Read the model definition and answer for the solid it produces. Units are mm, in the model's axes. A direction names the side the tool comes from. Give positions to 0.01 mm unless a question says otherwise; leave off trailing zeros. Order: outer loops, then holes, each group sorted by start corner. A loop starts at its lowest first (then second) coordinate and runs counter-clockwise, first axis right, second up. Notation, with made-up numbers: (58.5, 39.25) -> (111.5, 39.25) arc R31 ccw to (111.5, 71.25) -> close; hole circle Ø7 at (24, 57.25). An arc over 180 degrees is marked (long way). Answer as CSV lines item,"result". Start each with the question number.
1) The mould has two halves that part along Z. Classify faces 3 (the face through (9, 561, -218.338)), 4 (the face through (0, 295, -182)), 5 (the face through (9, 173, 0)): +Z half, -Z half, draft (parallel to the pull), parting line (faces both ways), or undercut.
2) Find section C-C (y = 425). Determine the outline of the cut face in (x, z), and give its area (3 significant figures).
3) Find section B-B (z = -304.5). Determine the outline of the cut face in (x, y).
4) Straight lines are drawn through the part: L1, parallel to Z at x = 15.5, y = 241.5; L2, parallel to Z at x = 5.75, y = 555; L3, parallel to Z at x = 5.5, y = 254. For each, find the intervals that lie inside material, in ascending order. Write a range as from..to.
5) Flat-ended cylindrical pins translate along their axes: pin 1 Ø5 at (x, y) = (13, 566) entering from +Z; pin 2 Ø1.5 at (x, y) = (15, 448) entering from -Z. Find the tip coordinate at first contact, or state that the pin passes through.
6) For faces 1 (the face through (9, 119, -368.3)), 2 (the face through (9, 562, -151.663)), determine the directions among +Z, -Z, +X, -X, +Y, -Y from which every point of the face is accessible in a straight line to the end or side of a thin tool.
7) Find section A-A (x = 5). Determine the outline of the cut face in (y, z) (1 decimal).
```python
from build123d import *

# Parameters (mm, degrees)
BOSS_EXTRUDE1_DEPTH = 17.4625
CUT_EXTRUDE1_DEPTH  = 17.4625
SKETCH2_R           = 3.96875
CUT_EXTRUDE2_DEPTH  = 17.4625


with BuildPart() as part:
    # Sketch1 → Boss-Extrude1 (new body)
    with BuildSketch(Plane(origin=(0, 0, 0), x_dir=(0, 0, -1), z_dir=(1, 0, 0))):
        Polygon((0, 0), (368.3, 0), (368.3, 241.3), (289.73584427, 581.598745126), (80.26426737, 581.598745126), (0, 340.614), align=None)
    extrude(amount=BOSS_EXTRUDE1_DEPTH)

    # RockerBoxCutout → Cut-Extrude1 (cut)
    with BuildSketch(Plane(origin=(17.4625, 0, 0), x_dir=(0, 0, -1), z_dir=(1, 0, 0))):
        with BuildLine():
            ThreePointArc((218.33755582, 541.911245126), (185.00005582, 575.248745126), (151.66255582, 541.911245126))
            Line((151.66255582, 541.911245126), (218.33755582, 541.911245126))
        make_face()
        with BuildLine():
            Line((218.33755582, 541.911245126), (151.66255582, 541.911245126))
            ThreePointArc((151.66255582, 541.911245126), (185.00005582, 508.573745126), (218.33755582, 541.911245126))
        make_face()
        with BuildLine():
            Line((151.66255582, 581.598745126), (151.66255582, 541.911245126))
            ThreePointArc((151.66255582, 541.911245126), (185.00005582, 575.248745126), (218.33755582, 541.911245126))
            Line((218.33755582, 541.911245126), (218.33755582, 581.598745126))
            Line((218.33755582, 581.598745126), (151.66255582, 581.598745126))
        make_face()
    extrude(amount=-CUT_EXTRUDE1_DEPTH, mode=Mode.SUBTRACT)

    # Sketch2 → Cut-Extrude2 (cut)
    with BuildSketch(Plane.ZY):
        with Locations((-13, 60)):
            Circle(SKETCH2_R)
        with Locations((-13, 290.1875)):
            Circle(SKETCH2_R)
    extrude(amount=-CUT_EXTRUDE2_DEPTH, mode=Mode.SUBTRACT)


solid = part.part
```
Findings below:
1,face 3,"undercut"
1,face 4,"draft"
1,face 5,"+Z half"
2,outline,"(0, -325.89) -> (17.46, -325.89) -> (17.46, -28.11) -> (0, -28.11) -> close"
2,area,"5,200 mm²"
3,outline,"(0, 0) -> (17.46, 0) -> (17.46, 517.65) -> (0, 517.65) -> close"
4,L1,"-368.25..0"
4,L2,"-295.88..-218.34, -151.66..-71.41"
4,L3,"-365.37..0"
5,pin 1,"z = -74.24"
5,pin 2,"z = -320.75"
6,face 1,"-Z, +X, -X, +Y, -Y"
6,face 2,"+X, -X, +Y"
7,outline,"(0, -368.3) -> (241.3, -368.3) -> (581.6, -289.7) -> (581.6, -218.3) -> (541.9, -218.3) arc R33.3 cw to (541.9, -151.7) -> (581.6, -151.7) -> (581.6, -80.3) -> (340.6, 0) -> (0, 0) -> close; hole circle Ø7.9 at (60, -13); hole circle Ø7.9 at (290.2, -13)"
